The figure shows three views and two pictorial views of one solid part (mm, origin at its lowest corner). Answer the questions. A direction names the side the tool comes from. Round coordinates to 2 decimals unless told otherwise and drop trailing zeros. Loops run counter-clockwise (first coordinate to the right, second up) from the corner with the lowest first, then second, coordinate; pieces in that order, holes last. Notation, with made-up numbers: (-34.75, 13.25) -> (-12.75, 13.25) arc R12 ccw to (-12.75, 23.25) -> close; hole circle Ø7 at (10, -1). An arc over 180 degrees is marked (long way). Put each result on its own line as item: value.
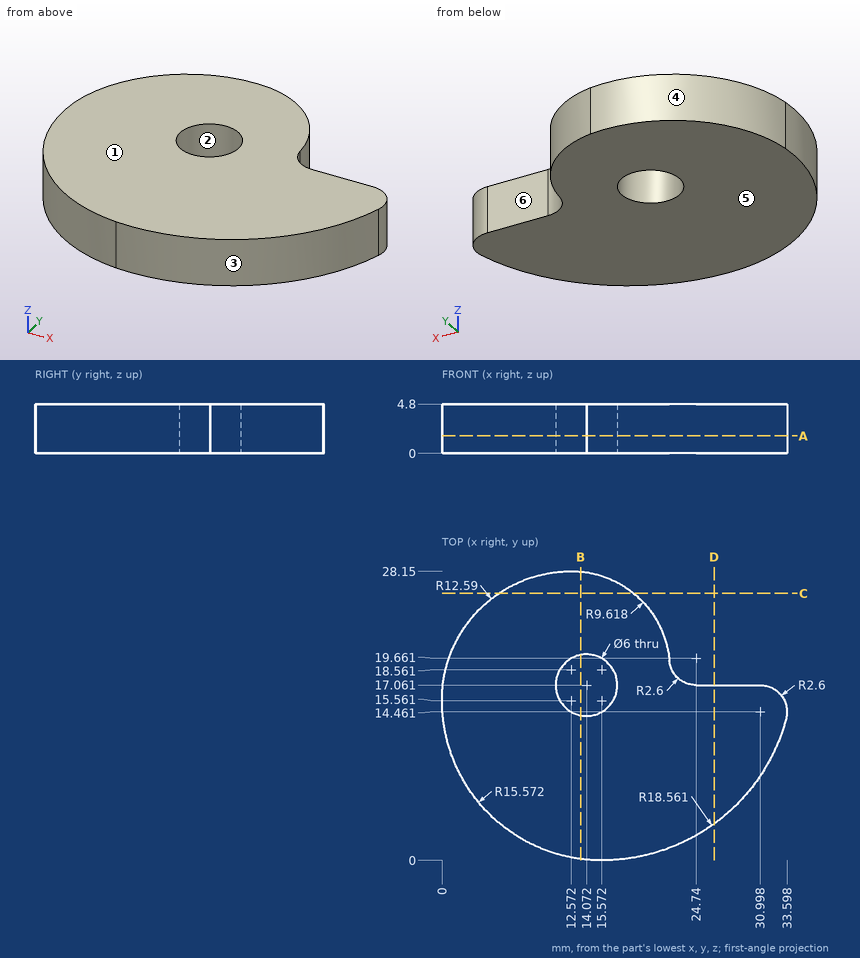
Item 1: The part is cut by section D-D (x = 26.5). Determine the outline of the cut face in (y, z), then the cut area to 3 significant figures.
Derived:
outline: (3.56, 0) -> (17.06, 0) -> (17.06, 4.8) -> (3.56, 4.8) -> close
area: 64.8 mm^2
Item 2: Which of the six approach directions +Z, -Z, +X, -X, +Y, -Y give full straight-line access (tool end or side, diameter ignored) to the marked faces 5 and 6?
Derived:
face 5: -Z, +X, -X, +Y, -Y
face 6: +Z, -Z, +X, +Y
Item 3: A flat-ended cylindrical pin translates along its axis: pin 1 Ø1.5 at (y, z) = (25, 2) entering from +X. Find the tip coordinate at first contact, or state that the pin passes through.
Derived:
pin 1: stops at x = 20.33
Item 4: The part is cut by section A-A (z = 1.7). Determine the outline of the cut face in (x, y) (1 decimal).
Derived:
outline: (0.1, 17.1) arc R15.6 ccw to (14.1, 0.1) arc R18.6 ccw to (33.5, 13.8) arc R2.6 ccw to (31, 17.1) -> (24.7, 17.1) arc R2.6 cw to (22.2, 19.4) arc R9.6 ccw to (14.1, 28.1) arc R12.6 ccw to start; hole circle Ø6 at (14.1, 17.1)
Item 5: The part is cut by section B-B (x = 13.5). Determine the outline of the cut face in (y, z) (1 decimal), then the cut area to 3 significant figures.
Derived:
outline: (0.1, 0) -> (14.1, 0) -> (14.1, 4.8) -> (0.1, 4.8) -> close; (20, 0) -> (28.1, 0) -> (28.1, 4.8) -> (20, 4.8) -> close
area: 106 mm^2
Item 6: The part is cut by section C-C (y = 26). Determine the outline of the cut face in (x, z) (1 decimal).
Derived:
outline: (5.5, 0) -> (18.7, 0) -> (18.7, 4.8) -> (5.5, 4.8) -> close
Item 7: Find the intervals of material crossed by line 1 along Y through (x, z) = (16, 3.7) (1 decimal); line 2 along X through (y, z) = (27, 4.3) (1 decimal); line 3 along Y through (x, z) = (27, 3.15) (1 decimal), in increasing order.
Derived:
line 1: y = 0 to 14.8, 19.4 to 27.5
line 2: x = 7.3 to 17.2
line 3: y = 3.9 to 17.1
Item 8: For a pull along Y with two mould halves and no side action, classify the marked faces 1, 2, 3 and 4 as pulls with the +Y half, pulls with the -Y half, needs draft (parallel to the pull), parting line crosses it, or undercut.
Derived:
face 1: needs draft
face 2: undercut
face 3: pulls with the -Y half
face 4: pulls with the +Y half
